Study the drawing (mm; zero at the part's minimum x, y, z) and answer. A direction names the side the tool comes from. Give positions to 0.01 mm unless a question says otherwise; leave off trailing zeros. Write each loop counter-clockwise with the first axis right and the second up, starting at its lowest first coordinate (ties: lowest second). Pieces come first, ordered by that corner, then holes.
1) Find section D-D (y = 61.5). Determine the outline of the cut face in (x, z), plus the area to 4 significant figures.
2) A tool of negligible diameter and unlimited length cuts with its end or side. For the marked faces 1 and 2, from which of +Z, -Z, +X, -X, +Y, -Y can it reach the whole face along a straight path? Write none if from no direction.
3) Find section C-C (y = 279.5). Determine the outline of the cut face in (x, z), plus the area to 3 significant figures.
4) Straight lines are drawn through the part: probe 1 along X at (y, z) = (47.5, 288.5); probe 2 along Z at (x, y) = (156, 151.5). For each, find the intervals that lie inside material, in ascending order.
5) Determine the mould class of the marked faces 3, 4, 5 and 6 for opening direction X: pulls with the +X half, pulls with the -X half, needs draft (parallel to the pull), parting line crosses it, or undercut.
6) Find section B-B (x = 235). Determine the outline of the cut face in (y, z).
7) Find section A-A (z = 191.5). Determine the outline of the cut face in (x, y).
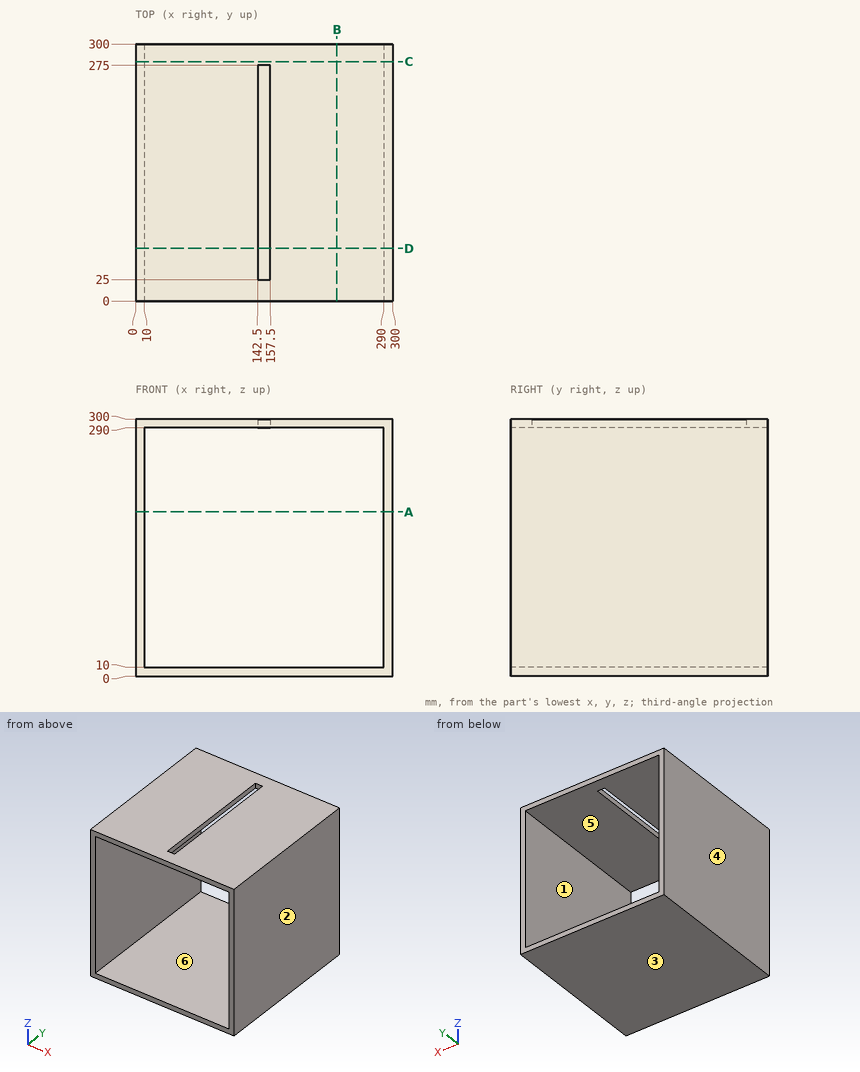
Results:
1. outline: (0, 0) - (300, 0) - (300, 300) - (157.5, 300) - (157.5, 290) - (290, 290) - (290, 10) - (10, 10) - (10, 290) - (142.5, 290) - (142.5, 300) - (0, 300) - close
1. area: 11,450 mm2
2. face 1: +Y, -Y
2. face 2: +Z, -Z, +X, +Y, -Y
3. outline: (0, 0) - (300, 0) - (300, 300) - (0, 300) - close; hole (10, 10) - (290, 10) - (290, 290) - (10, 290) - close
3. area: 11,600 mm2
4. probe 1: x = 0 to 10, 290 to 300
4. probe 2: z = 0 to 10
5. face 3: needs draft
5. face 4: pulls with the -X half
5. face 5: undercut
5. face 6: undercut
6. outline: (0, 0) - (300, 0) - (300, 10) - (0, 10) - close; (0, 290) - (300, 290) - (300, 300) - (0, 300) - close
7. outline: (0, 0) - (10, 0) - (10, 300) - (0, 300) - close; (290, 0) - (300, 0) - (300, 300) - (290, 300) - close
